Design review of the part built by this model. Coordinates are the model's own, in mm. Give positions to 0.01 mm unless a question says otherwise; leave off trailing zeros. Loops run counter-clockwise (first coordinate to the right, second up) from the corner with the lowest first, then second, coordinate; pieces in that order, holes last. Notation, with made-up numbers: (-33, -11) -> (-9, -11) arc R20 ccw to (-9, 2) -> close; hole circle Ø7 at (23.5, 81). An arc over 180 degrees is marked (long way). Use a Markdown table: item, result. Add a question column.
1. Add section B-B (x = -122.5). State the section outline as (y, z) points.
2. For pin 1 Ø6 at (x, y) = (-183.5, -56) entering from -Z; pin 2 Ø4.5 at (x, y) = (-332.5, -132.5) entering from +Z, all flat-tipped, find the tip position at first contact; note any pin that passes through.
3. Add section A-A (x = -245). State the section outline as (y, z) points.
4. To check wall thickness, follow line 1 (Y direction, x = -105, z = 0.6); line 2 (Y direction, x = -210, z = 2.3); line 3 (Y direction, x = 332.5, z = 1.8). State the ranges of each line that lie inside material, in increasing order.
5. Add section C-C (y = -90). Count the separate pieces of the cut face and the enclosed holes in it, and give its area (3 significant figures).
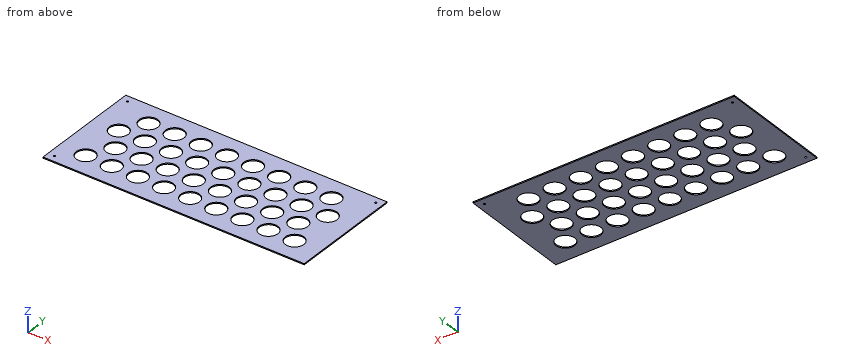
```python
from build123d import *

# Parameters (mm, degrees)
F0_W     = 700
F0_H     = 300
F0_R     = 2.5
F0_R_2   = 25
F1_DEPTH = 3


with BuildPart() as f1:
    # F0 (on Top) → F1 (new body)
    with BuildSketch(Plane.XY):
        Rectangle(F0_W, F0_H)
        with Locations((-332.5, -132.5)):
            Circle(F0_R, mode=Mode.SUBTRACT)
        with Locations((-280, -90)):
            Circle(F0_R_2, mode=Mode.SUBTRACT)
        with Locations((-210, -90)):
            Circle(F0_R_2, mode=Mode.SUBTRACT)
        with Locations((-140, -90)):
            Circle(F0_R_2, mode=Mode.SUBTRACT)
        with Locations((-70, -90)):
            Circle(F0_R_2, mode=Mode.SUBTRACT)
        with Locations((-245, -29.378222)):
            Circle(F0_R_2, mode=Mode.SUBTRACT)
        with Locations((-175, -29.378222)):
            Circle(F0_R_2, mode=Mode.SUBTRACT)
        with Locations((-105, -29.378222)):
            Circle(F0_R_2, mode=Mode.SUBTRACT)
        with Locations((-35, -29.378222)):
            Circle(F0_R_2, mode=Mode.SUBTRACT)
        with Locations((0, -90)):
            Circle(F0_R_2, mode=Mode.SUBTRACT)
        with Locations((70, -90)):
            Circle(F0_R_2, mode=Mode.SUBTRACT)
        with Locations((140, -90)):
            Circle(F0_R_2, mode=Mode.SUBTRACT)
        with Locations((210, -90)):
            Circle(F0_R_2, mode=Mode.SUBTRACT)
        with Locations((280, -90)):
            Circle(F0_R_2, mode=Mode.SUBTRACT)
        with Locations((35, -29.378222)):
            Circle(F0_R_2, mode=Mode.SUBTRACT)
        with Locations((105, -29.378222)):
            Circle(F0_R_2, mode=Mode.SUBTRACT)
        with Locations((175, -29.378222)):
            Circle(F0_R_2, mode=Mode.SUBTRACT)
        with Locations((245, -29.378222)):
            Circle(F0_R_2, mode=Mode.SUBTRACT)
        with Locations((-280, 30)):
            Circle(F0_R_2, mode=Mode.SUBTRACT)
        with Locations((-210, 30)):
            Circle(F0_R_2, mode=Mode.SUBTRACT)
        with Locations((-140, 30)):
            Circle(F0_R_2, mode=Mode.SUBTRACT)
        with Locations((-70, 30)):
            Circle(F0_R_2, mode=Mode.SUBTRACT)
        with Locations((-245, 90.621778)):
            Circle(F0_R_2, mode=Mode.SUBTRACT)
        with Locations((-332.5, 132.5)):
            Circle(F0_R, mode=Mode.SUBTRACT)
        with Locations((-175, 90.621778)):
            Circle(F0_R_2, mode=Mode.SUBTRACT)
        with Locations((-105, 90.621778)):
            Circle(F0_R_2, mode=Mode.SUBTRACT)
        with Locations((-35, 90.621778)):
            Circle(F0_R_2, mode=Mode.SUBTRACT)
        with Locations((0, 30)):
            Circle(F0_R_2, mode=Mode.SUBTRACT)
        with Locations((70, 30)):
            Circle(F0_R_2, mode=Mode.SUBTRACT)
        with Locations((140, 30)):
            Circle(F0_R_2, mode=Mode.SUBTRACT)
        with Locations((210, 30)):
            Circle(F0_R_2, mode=Mode.SUBTRACT)
        with Locations((280, 30)):
            Circle(F0_R_2, mode=Mode.SUBTRACT)
        with Locations((35, 90.621778)):
            Circle(F0_R_2, mode=Mode.SUBTRACT)
        with Locations((105, 90.621778)):
            Circle(F0_R_2, mode=Mode.SUBTRACT)
        with Locations((175, 90.621778)):
            Circle(F0_R_2, mode=Mode.SUBTRACT)
        with Locations((245, 90.621778)):
            Circle(F0_R_2, mode=Mode.SUBTRACT)
        with Locations((332.5, 132.5)):
            Circle(F0_R, mode=Mode.SUBTRACT)
    extrude(amount=F1_DEPTH)


solid = f1.part
```
Taken from the geometry:
| question | item | result |
|---|---|---|
| 1 | outline | (-150, 0) -> (-107.85, 0) -> (-107.85, 3) -> (-150, 3) -> close; (-72.15, 0) -> (-47.23, 0) -> (-47.23, 3) -> (-72.15, 3) -> close; (-11.52, 0) -> (12.15, 0) -> (12.15, 3) -> (-11.52, 3) -> close; (47.85, 0) -> (72.77, 0) -> (72.77, 3) -> (47.85, 3) -> close; (108.48, 0) -> (150, 0) -> (150, 3) -> (108.48, 3) -> close |
| 2 | pin 1 | stops at z = 0 |
| 2 | pin 2 | passes through |
| 3 | outline | (-150, 0) -> (-54.38, 0) -> (-54.38, 3) -> (-150, 3) -> close; (-4.38, 0) -> (65.62, 0) -> (65.62, 3) -> (-4.38, 3) -> close; (115.62, 0) -> (150, 0) -> (150, 3) -> (115.62, 3) -> close |
| 4 | line 1 | y = -150 to -54.38, -4.38 to 65.62, 115.62 to 150 |
| 4 | line 2 | y = -150 to -115, -65 to 5, 55 to 150 |
| 4 | line 3 | y = -150 to 130, 135 to 150 |
| 5 | separate pieces | 10 |
| 5 | enclosed holes | 0 |
| 5 | area | 750 mm^2 |
